The listing builds one solid part. Answer for the finished solid, in the listing's coordinates (mm). Coordinates: 2 decimals unless noted, no trailing zeros. Order: outer loops, then holes, each group sorted by start corner. A loop starts at its lowest first (then second) coordinate and runs counter-clockwise, first axis right, second up. Notation, with made-up numbers: (-30.5, -3.75) -> (6.5, -3.75) arc R29 ccw to (6.5, 30.25) -> close; hole circle Ø9 at (88, -7.5). An arc over 180 degrees is marked (long way). Return JSON: item names as keys, results as strings.
```python
from build123d import *

# Parameters (mm, degrees)
SKETCH1_R           = 1.6
BOSS_EXTRUDE1_DEPTH = 3


with BuildPart() as part:
    # Sketch1 → Boss-Extrude1 (new body)
    with BuildSketch(Plane(origin=(0, 0, 0), x_dir=(1, 0, 0), z_dir=(0, 1, 0))):
        Polygon((86.535317855, -129.61721435), (86.535317855, -119.61721435), (81.535317855, -114.61721435), (-33.464682145, -114.61721435), (-33.464682145, -195.61721435), (81.535317855, -195.61721435), (86.535317855, -190.61721435), (86.535317855, -180.61721435), align=None)
        with Locations((12.469945392, -125.100274039)):
            Circle(SKETCH1_R, mode=Mode.SUBTRACT)
        with Locations((-8.062851064, -128.720760043)):
            Circle(SKETCH1_R, mode=Mode.SUBTRACT)
        with Locations((-21.464682145, -144.692440382)):
            Circle(SKETCH1_R, mode=Mode.SUBTRACT)
        with Locations((-21.464682145, -165.541988319)):
            Circle(SKETCH1_R, mode=Mode.SUBTRACT)
        with Locations((-8.062851064, -181.513668658)):
            Circle(SKETCH1_R, mode=Mode.SUBTRACT)
        with Locations((12.469945392, -185.134154662)):
            Circle(SKETCH1_R, mode=Mode.SUBTRACT)
        Polygon((-18.464682145, -134.11721435), (6.535317855, -134.11721435), (6.535317855, -129.61721435), (70.535317855, -129.61721435), (75.535317855, -134.61721435), (75.535317855, -175.61721435), (70.535317855, -180.61721435), (6.535317855, -180.61721435), (6.535317855, -176.11721435), (-18.464682145, -176.11721435), align=None, mode=Mode.SUBTRACT)
    extrude(amount=BOSS_EXTRUDE1_DEPTH)


solid = part.part
```
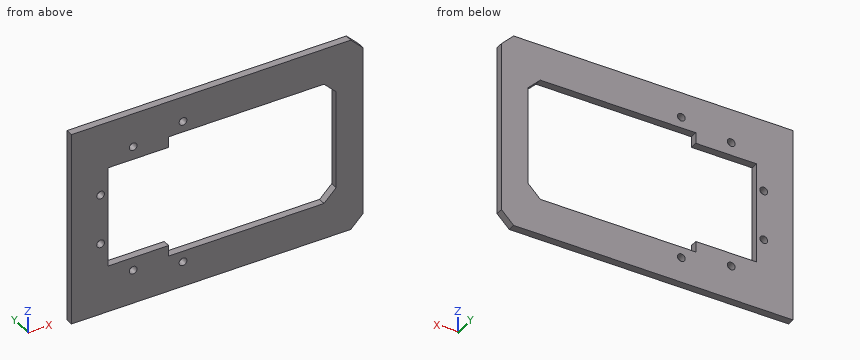
Item 1: The part is cut by section C-C on y = 0.45. Determine the outline of the cut face in (x, z).
Answer list:
{"outline": "(-33.46, 114.62) -> (81.54, 114.62) -> (86.54, 119.62) -> (86.54, 190.62) -> (81.54, 195.62) -> (-33.46, 195.62) -> close; hole circle Ø3.2 at (-21.46, 144.69); hole circle Ø3.2 at (-21.46, 165.54); hole (-18.46, 134.12) -> (6.54, 134.12) -> (6.54, 129.62) -> (70.54, 129.62) -> (75.54, 134.62) -> (75.54, 175.62) -> (70.54, 180.62) -> (6.54, 180.62) -> (6.54, 176.12) -> (-18.46, 176.12) -> close; hole circle Ø3.2 at (-8.06, 128.72); hole circle Ø3.2 at (-8.06, 181.51); hole circle Ø3.2 at (12.47, 125.1); hole circle Ø3.2 at (12.47, 185.13)"}
Item 2: The part is cut by section A-A on z = 160. Determine the outline of the cut face in (x, y), plus the area to 3 significant figures.
Answer list:
{"outline": "(-33.46, 0) -> (-18.46, 0) -> (-18.46, 3) -> (-33.46, 3) -> close; (75.54, 0) -> (86.54, 0) -> (86.54, 3) -> (75.54, 3) -> close", "area": "78.0 mm2"}
Item 3: A flat-ended cylindrical pin translates along its axis: pin 1 (2.5 mm diameter, centred on x = -8.06, z = 128.72, fed in from +Y). Find the tip coordinate at first contact, or state that the pin passes through.
Answer list:
{"pin 1": "through"}
Item 4: The part is cut by section B-B on x = 29.5. Determine the outline of the cut face in (y, z), plus the area to 3 significant figures.
Answer list:
{"outline": "(0, 114.62) -> (3, 114.62) -> (3, 129.62) -> (0, 129.62) -> close; (0, 180.62) -> (3, 180.62) -> (3, 195.62) -> (0, 195.62) -> close", "area": "90.0 mm2"}
Item 5: Find the intervals of material crossed by probe 1 along Z at (x, y) = (-16, 1.7); probe 2 along Z at (x, y) = (40, 1.85); probe 3 along X at (y, z) = (1.7, 155), in increasing order.
Answer list:
{"probe 1": "114.62 to 134.12, 176.12 to 195.62", "probe 2": "114.62 to 129.62, 180.62 to 195.62", "probe 3": "-33.46 to -18.46, 75.54 to 86.54"}
